from build123d import *

# Parameters (mm, degrees)
SKETCH2_R                = 4.3
SKETCH2_R_2              = 2.75
BOSS_EXTRUDE1_DEPTH      = 3
SKETCH3_R                = 4.3
SKETCH3_R_2              = 1.35
BOSS_EXTRUDE2_DEPTH      = 2.1
BOSS_EXTRUDE3_DEPTH      = 0.5
BOSS_EXTRUDE3_DEPTH_BACK = 2.1
SKETCH4_R                = 4.3
SKETCH4_R_2              = 0.25


with BuildPart() as part:
    # Sketch2 → Boss-Extrude1 (new body)
    with BuildSketch(Plane(origin=(0, 0, 0), x_dir=(1, 0, 0), z_dir=(0, 1, 0))):
        with Locations(Location((0, 0, 0), (0, 0, 270))):
            Circle(SKETCH2_R)
        with Locations(Location((0, 0, 0), (0, 0, 270))):
            Circle(SKETCH2_R_2, mode=Mode.SUBTRACT)
    extrude(amount=BOSS_EXTRUDE1_DEPTH)



with BuildPart() as body_2:
    # Sketch3 → Boss-Extrude2 (new body)
    with BuildSketch(Plane(origin=(0, 3, 0), x_dir=(1, 0, 0), z_dir=(0, 1, 0))):
        with Locations(Location((0, 0, 0), (0, 0, 270))):
            Circle(SKETCH3_R)
        with Locations(Location((0, 0, 0), (0, 0, 270))):
            Circle(SKETCH3_R_2, mode=Mode.SUBTRACT)
    extrude(amount=BOSS_EXTRUDE2_DEPTH)


with BuildPart() as part_1:
    add(part.part)

    add(body_2.part)  # Boss-Extrude3 merges body 2
    # Sketch4 → Boss-Extrude3 (add, two sides: drawn at the far end of the back side and taken through both)
    with BuildSketch(Plane(origin=(0, 5.1, 0), x_dir=(1, 0, 0), z_dir=(0, 1, 0)).offset(-BOSS_EXTRUDE3_DEPTH_BACK)):
        with BuildLine():
            Line((-2.030550566, 16.72355418), (-6.25525056, 1.766873065))
            ThreePointArc((-6.25525056, 1.766873065), (-6.5, 0), (-6.25525056, -1.766873065))
            Line((-6.25525056, -1.766873065), (-2.030550566, -16.72355418))
            ThreePointArc((-2.030550566, -16.72355418), (0, -18.26), (2.030550566, -16.72355418))
            Line((2.030550566, -16.72355418), (6.25525056, -1.766873065))
            ThreePointArc((6.25525056, -1.766873065), (6.5, 0), (6.25525056, 1.766873065))
            Line((6.25525056, 1.766873065), (2.030550566, 16.72355418))
            ThreePointArc((2.030550566, 16.72355418), (0, 18.26), (-2.030550566, 16.72355418))
        make_face()
        with Locations(Location((0, 0, 0), (0, 0, 270))):
            Circle(SKETCH4_R, mode=Mode.SUBTRACT)
        with Locations(Location((0, 16.15, 0), (0, 0, 270))):
            Circle(SKETCH4_R_2, mode=Mode.SUBTRACT)
        with Locations(Location((0, 13.15, 0), (0, 0, 270))):
            Circle(SKETCH4_R_2, mode=Mode.SUBTRACT)
        with Locations(Location((0, 10.15, 0), (0, 0, 270))):
            Circle(SKETCH4_R_2, mode=Mode.SUBTRACT)
        with Locations(Location((0, 7.15, 0), (0, 0, 270))):
            Circle(SKETCH4_R_2, mode=Mode.SUBTRACT)
        with Locations(Location((0, -7.15, 0), (0, 0, 90))):
            Circle(SKETCH4_R_2, mode=Mode.SUBTRACT)
        with Locations(Location((0, -10.15, 0), (0, 0, 90))):
            Circle(SKETCH4_R_2, mode=Mode.SUBTRACT)
        with Locations(Location((0, -13.15, 0), (0, 0, 90))):
            Circle(SKETCH4_R_2, mode=Mode.SUBTRACT)
        with Locations(Location((0, -16.15, 0), (0, 0, 90))):
            Circle(SKETCH4_R_2, mode=Mode.SUBTRACT)
    extrude(amount=BOSS_EXTRUDE3_DEPTH + BOSS_EXTRUDE3_DEPTH_BACK)


solid = part_1.part
Here's how the part is built. I have some questions about the finished solid (model axes, mm). A direction names the side the tool comes from. Coordinates: 2 decimals unless noted, no trailing zeros. Loops run counter-clockwise (first coordinate to the right, second up) from the corner with the lowest first, then second, coordinate; pieces in that order, holes last. Notation, with made-up numbers: (25, -37) -> (31, -37) arc R24 ccw to (31, -17) -> close; hole circle Ø8 at (30.25, 73.5). An arc over 180 degrees is marked (long way). Use one line per item in the form item = value. Start each with the question number.
(1) If we section it at A-A (y = 3.7): Give the number of separate pieces and of enclosed holes in the cut face, then the cut area to 3 significant figures.
(2) If we section it at B-B (x = 0.75): Please give me the cut outline in (y, z).
(3) If we section it at D-D (z = 15.5): Please give me the cut outline in (x, y).
(4) Will these pins go through, and if not, where does the flat tip stop? pin 1 (3 mm diameter, centred on x = -2.5, y = 2.5, fed in from -Z); pin 2 (3 mm diameter, centred on x = 1, z = 4, fed in from +Y); pin 3 (2.5 mm diameter, centred on x = 0, z = 0, fed in from +Y) (3 decimals); pin 4 (2 mm diameter, centred on y = 5, z = -4, fed in from -X).
(5) Please list where these lines run through material, in increasing order: line 1 along Y through (x, z) = (-2, -1); line 2 along Y through (x, z) = (2, 4); line 3 along X through (y, z) = (4.3, -13.15).
(6) If we section it at C-C (x = 3.5): Please give me the cut outline in (y, z), then the cut area to 3 significant figures.
(7) On a 3-axis mill with a long thin cutter (end or side, diameter ignored), from which of +Z, -Z, +X, -X, +Y, -Y can I reach the whole of each face in a straight line? I mean faces 1 (the face through (1.4, 5.6, -4.3)), 2 (the face through (-2, 5.1, 0)). Say none if no direction works.
(8) We'd pull the mould along X, two halves only. Please class faces 3 (the face through (-6.5, 4.3, 0)), 4 (the face through (-2.62, 1.48, -3.41)), 5 (the face through (-2.685, 1.479, -0.596)): pulls with the +X half, pulls with the -X half, needs draft (parallel to the pull), parting line crosses it, or undercut.
Verdict:
q1.separate_pieces = 1
q1.enclosed_holes = 9
q1.area = 295 mm²
q2.outline = (0, -4.23) -> (3, -4.23) -> (3, -18.12) -> (5.6, -18.12) -> (5.6, -4.23) -> (5.1, -4.23) -> (5.1, -1.12) -> (3, -1.12) -> (3, -2.65) -> (0, -2.65) -> close; (0, 2.65) -> (3, 2.65) -> (3, 1.12) -> (5.1, 1.12) -> (5.1, 4.23) -> (5.6, 4.23) -> (5.6, 18.12) -> (3, 18.12) -> (3, 4.23) -> (0, 4.23) -> close
q3.outline = (-2.38, 3) -> (2.38, 3) -> (2.38, 5.6) -> (-2.38, 5.6) -> close
q4.pin_1 = -17.96
q4.pin_2 = 5.6
q4.pin_3 = through
q4.pin_4 = -5.91
q5.line_1 = 3 to 5.1
q5.line_2 = 3 to 5.6
q5.line_3 = -3.04 to -0.25, 0.25 to 3.04
q6.outline = (0, -2.5) -> (3, -2.5) -> (3, -11.52) -> (5.6, -11.52) -> (5.6, -2.5) -> (5.1, -2.5) -> (5.1, 2.5) -> (5.6, 2.5) -> (5.6, 11.52) -> (3, 11.52) -> (3, 2.5) -> (0, 2.5) -> close
q6.area = 72.4 mm²
q7.face_1 = +Z, -Z, +X, -X, +Y
q7.face_2 = +Y
q8.face_3 = pulls with the -X half
q8.face_4 = parting line crosses it
q8.face_5 = undercut
